```python
from build123d import *

# Parameters (mm, degrees)
F0_R     = 27.7491203527
F1_DEPTH = 93.98
F2_R     = 20.2221650078
F3_DEPTH = 34.036
F5_DEPTH = 50.8
F6_R     = 8.255
F8_DEPTH = 38.1


# Not quite as in the source:
# - the program builds the solid bodies; features that only make, move or delete a surface that nothing else refers to are left out


with BuildPart() as f1:
    # F0 (on Front) → F1 (new body)
    with BuildSketch(Plane.XZ):
        Circle(F0_R)
    extrude(amount=-F1_DEPTH)

    # F2 (on face) → F3 (join)
    with BuildSketch(Plane(origin=(0, 93.98, 0), x_dir=(-1, 0, 0), z_dir=(0, 1, 0))):
        Circle(F2_R)
    extrude(amount=F3_DEPTH)

    # F4 (on Front) → F5 (join)
    with BuildSketch(Plane.XZ):
        Polygon((-6.6853386185, -5.4466079127), (-6.6853386185, 0), (-6.6853386185, 14.8733920873), (-15.5753386185, 14.8733920873), (-15.5753386185, -5.4466079127), align=None)
        Polygon((9.04710629, 14.8733920873), (9.04710629, 0), (9.04710629, -5.4466079127), (17.93710629, -5.4466079127), (17.93710629, 14.8733920873), align=None)
    extrude(amount=F5_DEPTH)

    # F6 (on Right) → F8 (cut, symmetric)
    with BuildSketch(Plane.YZ):
        with Locations((-38.159750402, 4.5024077408)):
            Circle(F6_R)
    extrude(amount=F8_DEPTH, both=True, mode=Mode.SUBTRACT)


solid = f1.part
```
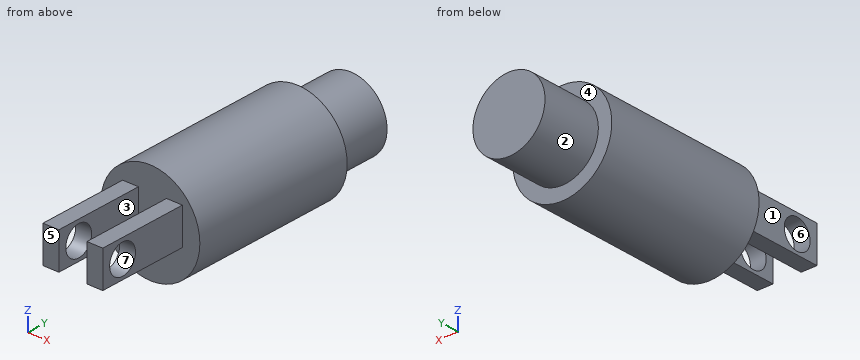
The listing builds one solid part. Answer for the finished solid, in the listing's coordinates (mm). Face numbers are marked on the shaded views. A direction names the side the tool comes from. Round coordinates to 2 decimals unless told otherwise and drop trailing zeros. Order: outer loops, then holes, each group sorted by start corner. A loop starts at its lowest first (then second) coordinate and runs counter-clockwise, first axis right, second up. Notation, with made-up numbers: (47.25, 51.25) -> (51.25, 51.25) arc R7 cw to (51.25, 64.25) -> close; hole circle Ø5 at (27.5, 63.5). An arc over 180 degrees is marked (long way). Answer as CSV lines item,"result". Start each with the question number.
(1) The part is cut by section C-C (z = 6.5). Determine the outline of the cut face in (x, y).
(2) For a pull along Y with two mould halves and no side action, classify the marked faces 4, 5, 6 and 7 as +Y half, -Y half, draft (parallel to the pull), parting line (faces both ways), or undercut.
(3) Find the intervals of material crossed by probe 1 along Z at (x, y) = (-8, -5); probe 2 along X at (y, z) = (34, -1); probe 3 along Y at (x, z) = (25, 11), in increasing order. Write a range as from..to.
(4) Flat-ended cylindrical pins translate along their axes: pin 1 Ø3 at (x, y) = (10, 93.5) entering from +Z; pin 2 Ø8 at (x, y) = (-18, 12) entering from -Z; pin 3 Ø10 at (y, z) = (-38.16, 4.5) entering from -X; pin 4 Ø22.5 at (y, z) = (-37.5, 1) entering from -X. Find the tip coordinate at first contact, or state that the pin passes through.
(5) A tool of negligible diameter and unlimited length cuts with its end or side. For the marked faces 1, 2 and 3, from which of +Z, -Z, +X, -X, +Y, -Y can it reach the whole face along a straight path? Write none if from no direction.
(6) The part is cut by section B-B (x = 0). Determine the outline of the cut face in (y, z).
(7) The part is cut by section A-A (y = -2). Determine the outline of the cut face in (x, z).
(8) The part is cut by section D-D (x = 11). Determine the outline of the cut face in (y, z) (3 decimals).
Evaluation:
1,outline,"(-26.98, 0) -> (-15.58, 0) -> (-15.58, -30.15) -> (-6.69, -30.15) -> (-6.69, 0) -> (9.05, 0) -> (9.05, -30.15) -> (17.94, -30.15) -> (17.94, 0) -> (26.98, 0) -> (26.98, 93.98) -> (19.15, 93.98) -> (19.15, 128.02) -> (-19.15, 128.02) -> (-19.15, 93.98) -> (-26.98, 93.98) -> close; (-15.58, -50.8) -> (-6.69, -50.8) -> (-6.69, -46.17) -> (-15.58, -46.17) -> close; (9.05, -50.8) -> (17.94, -50.8) -> (17.94, -46.17) -> (9.05, -46.17) -> close"
2,face 4,"+Y half"
2,face 5,"-Y half"
2,face 6,"undercut"
2,face 7,"undercut"
3,probe 1,"-5.45..14.87"
3,probe 2,"-27.73..27.73"
3,probe 3,"0..93.98"
4,pin 1,"z = 26.42"
4,pin 2,"z = -23.96"
4,pin 3,"through"
4,pin 4,"x = -15.58"
5,face 1,"+Z, -Z, -X, -Y"
5,face 2,"+Y"
5,face 3,"+Z, -Z, -Y"
6,outline,"(0, -27.75) -> (93.98, -27.75) -> (93.98, -20.22) -> (128.02, -20.22) -> (128.02, 20.22) -> (93.98, 20.22) -> (93.98, 27.75) -> (0, 27.75) -> close"
7,outline,"(-15.58, -5.45) -> (-6.69, -5.45) -> (-6.69, 14.87) -> (-15.58, 14.87) -> close; (9.05, -5.45) -> (17.94, -5.45) -> (17.94, 14.87) -> (9.05, 14.87) -> close"
8,outline,"(-50.8, -5.447) -> (0, -5.447) -> (0, -25.476) -> (93.98, -25.476) -> (93.98, -16.969) -> (128.016, -16.969) -> (128.016, 16.969) -> (93.98, 16.969) -> (93.98, 25.476) -> (0, 25.476) -> (0, 14.873) -> (-50.8, 14.873) -> close; hole circle Ø16.51 at (-38.16, 4.502)"
